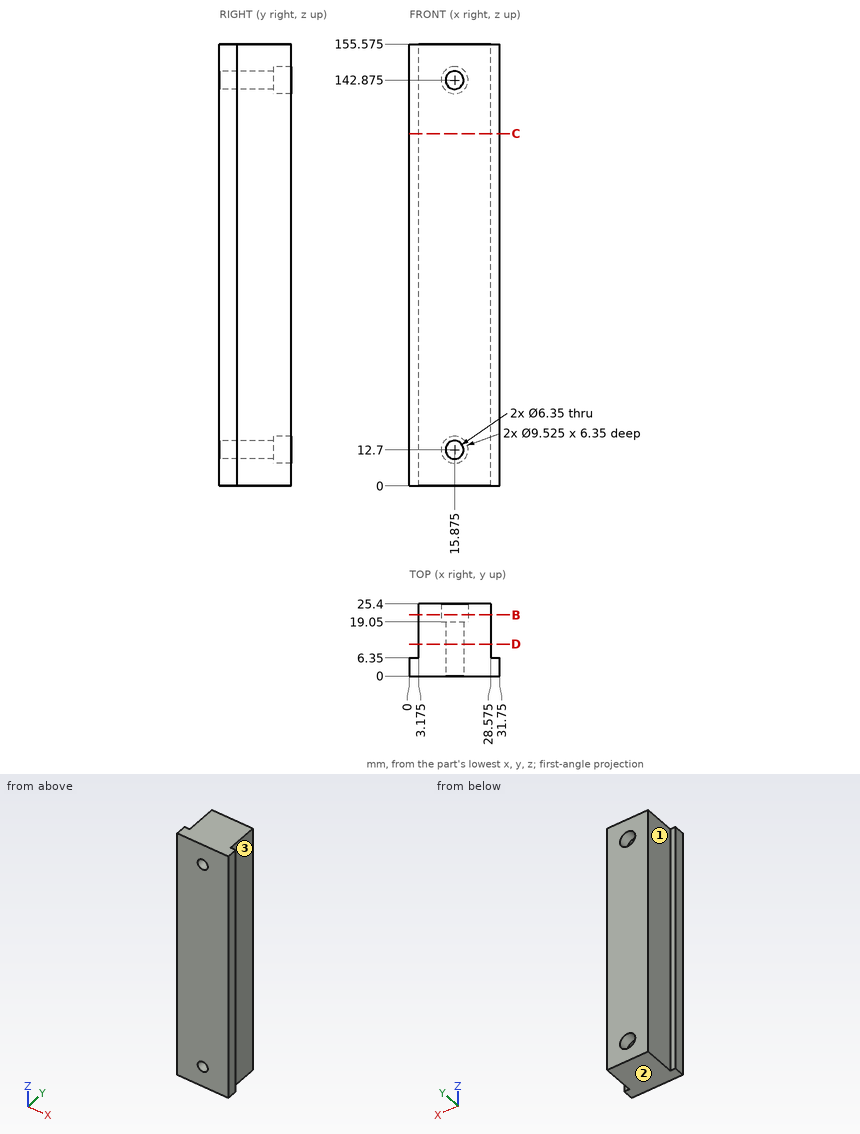
Geometry: see drawing. Coordinates: mm, zero at the bounding-box minimum. A direction names the side the tool comes from. Coordinates: 2 decimals unless noted, no trailing zeros. Order: outer loops, then holes, each group sorted by start corner. A loop starts at its lowest first (then second) coordinate and runs counter-clockwise, first axis right, second up. Notation, with made-up numbers: (-40, 17.25) - (18, 17.25) arc R32 ccw to (18, 50.25) - close; hole circle Ø3 at (48.5, 52). An arc over 180 degrees is marked (long way). Use one line per item in the form item = value.
1) Pin query (flat end, axial travel): pin 1 (11 mm diameter, centred on x = 15.875, z = 142.875, fed in from -Y); pin 2 (12 mm diameter, centred on y = 15, z = 57.5, fed in from -X) (3 decimals); pin 3 (9.5 mm diameter, centred on y = 11.5, z = 81.5, fed in from +X) (3 decimals); pin 4 (1 mm diameter, centred on x = 1, z = 76.5, fed in from +Y). Return the tip coordinate at first contact, or that it passes through.
Solutions:
pin_1 = 0
pin_2 = 3.175
pin_3 = 28.575
pin_4 = 6.35
2) Set-up query: the marked faces 1, 2 and 3. Return all of +Z, -Z, +X, -X, +Y, -Y with unobstructed straight access to the full face (end or side cutting, diameter ignored); none if empty.
Solutions:
face_1 = +Z, -Z, -X, +Y
face_2 = -Z, +X, -X, +Y, -Y
face_3 = +Z, -Z, +X, +Y
3) Section C-C (z = 124). Return loops of the section in (x, y) (3 decimals), then the cut area to 3 significant figures.
Solutions:
outline = (0, 0) - (31.75, 0) - (31.75, 6.35) - (28.575, 6.35) - (28.575, 25.4) - (3.175, 25.4) - (3.175, 6.35) - (0, 6.35) - close
area = 685 mm^2
4) Section D-D (y = 11.25). Return loops of the section in (x, z) (3 decimals), then the cut area to 3 significant figures.
Solutions:
outline = (3.175, 0) - (28.575, 0) - (28.575, 155.575) - (3.175, 155.575) - close; hole circle Ø6.35 at (15.875, 12.7); hole circle Ø6.35 at (15.875, 142.875)
area = 3,890 mm^2
5) Ray query, L1, parallel to Z at x = 16, y = 20 (3 decimals); L2, parallel to Z at x = 16, y = 14 (3 decimals); L3, parallel to X at y = 11.75, z = 12.7 (3 decimals). Return the intervals inside material, ascending.
Solutions:
L1 = 0 to 7.939, 17.461 to 138.114, 147.636 to 155.575
L2 = 0 to 9.527, 15.873 to 139.702, 146.048 to 155.575
L3 = 3.175 to 12.7, 19.05 to 28.575
6) Section B-B (y = 21.5). Return loops of the section in (x, z) (1 decimal).
Solutions:
outline = (3.2, 0) - (28.6, 0) - (28.6, 155.6) - (3.2, 155.6) - close; hole circle Ø9.5 at (15.9, 12.7); hole circle Ø9.5 at (15.9, 142.9)
